from build123d import *

# Parameters (mm, degrees)
SKETCH_1_W          = 14
SKETCH_1_H          = 14
EXTRUDE_1_DEPTH     = 14
SKETCH_2_W          = 10
SKETCH_2_H          = 10
SKETCH_2_R          = 3.9
EXTRUDE_2_DEPTH     = 4
SKETCH_3_R          = 5.4
CUT_EXTRUDE_1_DEPTH = 14


with BuildPart() as part:
    # 草图1 → 凸台-拉伸1 (new body)
    with BuildSketch(Plane(origin=(0, 0, 0), x_dir=(1, 0, 0), z_dir=(0, 1, 0))):
        with Locations((7, 7)):
            Rectangle(SKETCH_1_W, SKETCH_1_H)
    extrude(amount=EXTRUDE_1_DEPTH)

    # 草图2 → 凸台-拉伸2 (add)
    with BuildSketch(Plane.XY):
        with Locations((7, 7)):
            Rectangle(SKETCH_2_W, SKETCH_2_H)
        with Locations((7, 7)):
            Circle(SKETCH_2_R, mode=Mode.SUBTRACT)
    extrude(amount=EXTRUDE_2_DEPTH)

    # 草图3 → 切除-拉伸1 (cut)
    with BuildSketch(Plane(origin=(0, 14, 0), x_dir=(1, 0, 0), z_dir=(0, 1, 0))):
        with Locations(Location((7, 7, 0), (0, 0, 270))):
            Circle(SKETCH_3_R)
    extrude(amount=-CUT_EXTRUDE_1_DEPTH, mode=Mode.SUBTRACT)


solid = part.part
Work out the finished part from the listing and answer in its coordinate system (mm). A direction names the side the tool comes from. Round coordinates to 2 decimals unless told otherwise and drop trailing zeros. Order: outer loops, then holes, each group sorted by start corner. A loop starts at its lowest first (then second) coordinate and runs counter-clockwise, first axis right, second up. Notation, with made-up numbers: M 69.25,83 L 111.25,83 A24 ccw 111.25,118 Z; hole C 62.5,16 d6. An arc over 180 degrees is marked long. Put each result on its own line as item: value. Start each with the question number.
Q1. For a pull along X with two mould halves and no side action, classify faces 6 (the flat face through (1, 7, 0)), 7 (the flat face through (7, 7, 0)), 8 (the flat face through (12, 7, 2)) as pulls with the +X half, pulls with the -X half, needs draft (parallel to the pull), parting line crosses it, or undercut.
Q2. Section D-D, the plane z = 1.5 is taken. Write down the section's boundary in (x, y), and give its area (3 significant figures).
Q3. Section C-C, the plane x = 7 is taken. Write down the section's boundary in (y, z).
Q4. Straight lines are drawn through the part: L1, parallel to Y at x = 7, z = 2.25; L2, parallel to X at y = 4, z = -7; L3, parallel to Y at x = 11.5, z = 1.5. For each, find the intervals that lie inside material, in ascending order. Write a range as [from, to].
Q5. Section B-B, the plane z = -7 is taken. Write down the section's boundary in (x, y), and give its area (3 significant figures).
Q6. Section A-A, the plane y = 5.5 is taken. Write down the section's boundary in (x, z), and give its area (3 significant figures).
Q7. Flat-ended cylindrical pins translate along their axes: pin 1 (3 mm diameter, centred on y = 5.5, z = 2.5, fed in from +X); pin 2 (4 mm diameter, centred on x = 6, y = 9, fed in from +Z); pin 3 (5 mm diameter, centred on x = 6, z = -7.5, fed in from -Y); pin 4 (2 mm diameter, centred on x = 6, z = 1.5, fed in from +Y). Find the tip coordinate at first contact, or state that the pin passes through.
Q8. A tool of negligible diameter and unlimited length cuts with its end or side. For faces 1 (the cylindrical face through (9.097, 10.288, 1.972)), 2 (the flat face through (10, 0, -12)), 3 (the flat face through (7, 12, 2)), 4 (the flat face through (7, 2, 2)), 5 (the flat face through (2, 7, 2)), from which of +Z, -Z, +X, -X, +Y, -Y can it reach the whole face along a straight path? Write none if from no direction.
Findings below:
1. face 6: needs draft
1. face 7: undercut
1. face 8: pulls with the +X half
2. outline: M 2,2 L 12,2 L 12,12 L 2,12 Z; hole C 7,7 d7.8
2. area: 52.2 mm^2
3. outline: M 0,-14 L 14,-14 L 14,-12.4 L 0,-12.4 Z; M 0,-1.6 L 14,-1.6 L 14,0 L 12,0 L 12,4 L 10.9,4 L 10.9,0 L 3.1,0 L 3.1,4 L 2,4 L 2,0 L 0,0 Z
4. L1: y = [2, 3.1], [10.9, 12]
4. L2: x = [0, 1.6], [12.4, 14]
4. L3: y = [2, 12]
5. outline: M 0,0 L 1.6,0 L 1.6,14 L 0,14 Z; M 12.4,0 L 14,0 L 14,14 L 12.4,14 Z
5. area: 44.8 mm^2
6. outline: M 0,-14 L 14,-14 L 14,0 L 12,0 L 12,4 L 10.6,4 L 10.6,0 L 3.4,0 L 3.4,4 L 2,4 L 2,0 L 0,0 Z; hole C 7,-7 d10.8
6. area: 116 mm^2
7. pin 1: stops at x = 12
7. pin 2: stops at z = 4
7. pin 3: passes through
7. pin 4: stops at y = 12
8. face 1: +Z
8. face 2: +Z, -Z, +X, -X, -Y
8. face 3: +Z, +X, -X, +Y
8. face 4: +Z, +X, -X, -Y
8. face 5: +Z, -X, +Y, -Y
